Geometry check sheet. Reference: the model listing, model coordinates, mm. Face numbers are marked on the shaded views. Coordinates: 2 decimals unless noted, no trailing zeros. Order: outer loops, then holes, each group sorted by start corner. A loop starts at its lowest first (then second) coordinate and runs counter-clockwise, first axis right, second up. Notation, with made-up numbers: (-23, 31.5) -> (24, 31.5) arc R28 ccw to (24, 67.5) -> close; hole circle Ø1 at (-27, 73). An arc over 180 degrees is marked (long way). Answer as CSV lines item,"result". Start each with the question number.
from build123d import *

# Parameters (mm, degrees)
SKETCH1_R           = 10
BOSS_EXTRUDE1_DEPTH = 6.36
SKETCH2_R           = 1.15
CUT_EXTRUDE1_DEPTH  = 6.36
CUT_EXTRUDE2_REACH  = 17.506
SKETCH3_R           = 0.85
CUT_EXTRUDE3_REACH  = 17.506
SKETCH4_R           = 0.85


with BuildPart() as part:
    # Sketch1 → Boss-Extrude1 (new body)
    with BuildSketch(Plane(origin=(0, 0, 0), x_dir=(1, 0, 0), z_dir=(0, 1, 0))):
        with Locations(Location((0, 0, 0), (0, 0, 90))):
            Circle(SKETCH1_R)
    extrude(amount=BOSS_EXTRUDE1_DEPTH)

    # Sketch2 → Cut-Extrude1 (cut)
    with BuildSketch(Plane(origin=(0, 6.36, 0), x_dir=(1, 0, 0), z_dir=(0, 1, 0))):
        with Locations(Location((0, 0, 0), (0, 0, 270))):
            Circle(SKETCH2_R)
    extrude(amount=-CUT_EXTRUDE1_DEPTH, mode=Mode.SUBTRACT)

    # Sketch3 → Cut-Extrude2 (cut, up to next)
    with BuildSketch(Plane(origin=(0, 6.36, 0), x_dir=(1, 0, 0), z_dir=(0, 1, 0)), mode=Mode.PRIVATE) as cut_extrude2_sk1:
        with Locations(Location((4.959818651, -5.559019603, 0), (0, 0, 270))):
            Circle(SKETCH3_R)
    cut_extrude2_tool1 = extrude(cut_extrude2_sk1.sketch, amount=-CUT_EXTRUDE2_REACH, mode=Mode.PRIVATE) & part.part
    add(cut_extrude2_tool1.solids().sort_by_distance((4.959819, 6.36, 5.55902))[0], mode=Mode.SUBTRACT)

    # Sketch4 → Cut-Extrude3 (cut, up to next)
    with BuildSketch(Plane(origin=(0, 6.36, 0), x_dir=(1, 0, 0), z_dir=(0, 1, 0)), mode=Mode.PRIVATE) as cut_extrude3_sk1:
        with Locations(Location((-4.959818651, 5.559019603, 0), (0, 0, 270))):
            Circle(SKETCH4_R)
    cut_extrude3_tool1 = extrude(cut_extrude3_sk1.sketch, amount=-CUT_EXTRUDE3_REACH, mode=Mode.PRIVATE) & part.part
    add(cut_extrude3_tool1.solids().sort_by_distance((-4.959819, 6.36, -5.55902))[0], mode=Mode.SUBTRACT)


solid = part.part
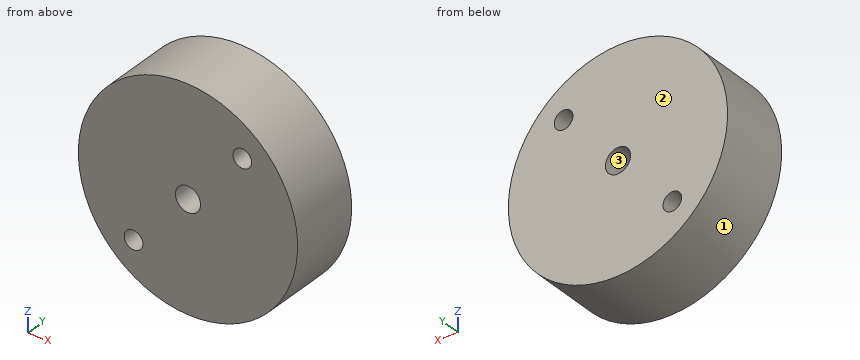
Q1. Thickness scan on L1, parallel to X at y = 3.25, z = 0; L2, parallel to Z at x = 5.25, y = 5.75; L3, parallel to Z at x = 5, y = 1. Record the ranges inside material, lowest first.
Q2. Sectioned sample at B-B, the plane z = 0. Record the cut outline in (x, y).
Q3. Release check for a two-part mould opening along Z. For the marked faces 1, 2 and 3 record: released by +Z, released by -Z, zero draft, split by the parting line, or undercut.
Q4. Go/stop test with flat-tipped pins: pin 1 Ø1 at (x, y) = (-4.5, 4) entering from +Z; pin 2 Ø2.5 at (x, z) = (-4.96, -5.56) entering from -Y; pin 3 Ø2 at (x, z) = (0, 0) entering from -Y; pin 4 Ø1.5 at (x, y) = (4, 2.5) entering from -Z. Record where each tip stops, or that it passes through.
Q5. Sectioned sample at D-D, the plane x = 3.5. Record the cut outline in (y, z).
Q6. Sectioned sample at C-C, the plane y = 3. Record the cut outline in (x, z), then the cut area to 3 significant figures.
Q7. Sectioned sample at A-A, the plane x = 0. Record the cut outline in (y, z), then the cut area to 3 significant figures.
Geometry results:
1,L1,"x = -10 to -1.15, 1.15 to 10"
1,L2,"z = -8.51 to 4.76, 6.36 to 8.51"
1,L3,"z = -8.66 to 4.71, 6.41 to 8.66"
2,outline,"(-10, 0) -> (-1.15, 0) -> (-1.15, 6.36) -> (-10, 6.36) -> close; (1.15, 0) -> (10, 0) -> (10, 6.36) -> (1.15, 6.36) -> close"
3,face 1,"split by the parting line"
3,face 2,"zero draft"
3,face 3,"undercut"
4,pin 1,"stops at z = 9.17"
4,pin 2,"stops at y = 0"
4,pin 3,"passes through"
4,pin 4,"stops at z = -9.46"
5,outline,"(0, -9.37) -> (6.36, -9.37) -> (6.36, 9.37) -> (0, 9.37) -> close"
6,outline,"circle Ø20 at (0, 0); hole circle Ø1.7 at (-4.96, -5.56); hole circle Ø2.3 at (0, 0); hole circle Ø1.7 at (4.96, 5.56)"
6,area,"305 mm^2"
7,outline,"(0, -10) -> (6.36, -10) -> (6.36, -1.15) -> (0, -1.15) -> close; (0, 1.15) -> (6.36, 1.15) -> (6.36, 10) -> (0, 10) -> close"
7,area,"113 mm^2"
